```python
from build123d import *

# Parameters (mm, degrees)
TRAY_START                        = 4.75
SKETCH1_W                         = 36.8
SKETCH1_H                         = 53.4
TRAY_DEPTH                        = 2.89
GROOVE_START                      = 7.14
SKETCH2_W                         = 34.6
SKETCH2_H                         = 53.2
GROOVE_DEPTH                      = 0.6
GROOVE_START_2                    = 6.6
SKETCH3_W                         = 34.6
SKETCH3_H                         = 10.45
GROOVE_PROTECTION_BOARD_END_DEPTH = 0.55
S1_S3_START                       = 4.65
SKETCH4_W                         = 9.25
SKETCH4_H                         = 6.5
SKETCH4_W_2                       = 9.05
S1_S3_AND_PLUGS_DEPTH             = 3.09
J4_START                          = 4.65
SKETCH5_W                         = 17.5
SKETCH5_H                         = 6
J4_AND_ITS_FLEX_DEPTH             = 3.09
ARM_START                         = 4.75
SKETCH6_W                         = 8
SKETCH6_H                         = 14.2
ARM_DEPTH                         = 1.5
BOARD_START                       = 1.6
SKETCH7_R                         = 2
BOARD_SCREW_FOOT_DEPTH            = 3.16
BOARD_START_2                     = 1.5
SKETCH8_R                         = 1.1
BOARD_SCREW_HOLE_DEPTH            = 6.24
BOARD_START_3                     = 5.94
SKETCH9_R                         = 1.95
BOARD_SCREW_COUNTERBORE_DEPTH     = 1.8
MIC_START                         = 1.8
SKETCH10_R                        = 1.5
MIC_TUBE_DEPTH                    = 2.96
MIC_START_2                       = 1.7
SKETCH11_R                        = 0.5
MIC_BORE_DEPTH                    = 4.3
MIC_START_3                       = 5
SKETCH12_W                        = 3.68
SKETCH12_H                        = 1
MIC_DUCT_DEPTH                    = 1
SNAP_START                        = -3
SNAP_DEPTH                        = 6


with BuildPart() as part:
    # Sketch1 → Tray (new body)
    with BuildSketch(Plane(origin=(0, 0, 0), x_dir=(1, 0, 0), z_dir=(0, 1, 0)).offset(TRAY_START)):
        with Locations((0, 5.95)):
            Rectangle(SKETCH1_W, SKETCH1_H)
    extrude(amount=TRAY_DEPTH)

    # Sketch2 → Groove (cut)
    with BuildSketch(Plane(origin=(0, 0, 0), x_dir=(1, 0, 0), z_dir=(0, 1, 0)).offset(GROOVE_START)):
        with Locations((0, 5.95)):
            Rectangle(SKETCH2_W, SKETCH2_H)
    extrude(amount=GROOVE_DEPTH, mode=Mode.SUBTRACT)

    # Sketch3 → Groove, protection-board end (cut)
    with BuildSketch(Plane(origin=(0, 0, 0), x_dir=(1, 0, 0), z_dir=(0, 1, 0)).offset(GROOVE_START_2)):
        with Locations((0, 27.325)):
            Rectangle(SKETCH3_W, SKETCH3_H)
    extrude(amount=GROOVE_PROTECTION_BOARD_END_DEPTH, mode=Mode.SUBTRACT)

    # Sketch4 → S1-S3 and plugs (cut)
    with BuildSketch(Plane(origin=(0, 0, 0), x_dir=(1, 0, 0), z_dir=(0, 1, 0)).offset(S1_S3_START)):
        with Locations((-13.825, 1.5)):
            Rectangle(SKETCH4_W, SKETCH4_H)
        with Locations((13.925, 20.57)):
            Rectangle(SKETCH4_W_2, SKETCH4_H)
        with Locations((13.825, -17.5)):
            Rectangle(SKETCH4_W, SKETCH4_H)
    extrude(amount=S1_S3_AND_PLUGS_DEPTH, mode=Mode.SUBTRACT)

    # Sketch5 → J4 and its flex (cut)
    with BuildSketch(Plane(origin=(0, 0, 0), x_dir=(1, 0, 0), z_dir=(0, 1, 0)).offset(J4_START)):
        with Locations((-0.35, 29.8)):
            Rectangle(SKETCH5_W, SKETCH5_H)
    extrude(amount=J4_AND_ITS_FLEX_DEPTH, mode=Mode.SUBTRACT)

    # Sketch6 → Arm (add)
    with BuildSketch(Plane(origin=(0, 0, 0), x_dir=(1, 0, 0), z_dir=(0, 1, 0)).offset(ARM_START)):
        with Locations((0, -27.7)):
            Rectangle(SKETCH6_W, SKETCH6_H)
    extrude(amount=ARM_DEPTH)

    # Sketch7 → Board screw foot (add)
    with BuildSketch(Plane(origin=(0, 0, 0), x_dir=(1, 0, 0), z_dir=(0, 1, 0)).offset(BOARD_START)):
        with Locations(Location((-15.64, 6.64, 0), (0, 0, 289.091052509))):
            Circle(SKETCH7_R)
    extrude(amount=BOARD_SCREW_FOOT_DEPTH)

    # Sketch8 → Board screw hole (cut)
    with BuildSketch(Plane(origin=(0, 0, 0), x_dir=(1, 0, 0), z_dir=(0, 1, 0)).offset(BOARD_START_2)):
        with Locations(Location((-15.64, 6.64, 0), (0, 0, 90))):
            Circle(SKETCH8_R)
    extrude(amount=BOARD_SCREW_HOLE_DEPTH, mode=Mode.SUBTRACT)

    # Sketch9 → Board screw counterbore (cut)
    with BuildSketch(Plane(origin=(0, 0, 0), x_dir=(1, 0, 0), z_dir=(0, 1, 0)).offset(BOARD_START_3)):
        with Locations((-15.64, 6.64)):
            Circle(SKETCH9_R)
    extrude(amount=BOARD_SCREW_COUNTERBORE_DEPTH, mode=Mode.SUBTRACT)

    # Sketch10 → Mic tube (add)
    with BuildSketch(Plane(origin=(0, 0, 0), x_dir=(1, 0, 0), z_dir=(0, 1, 0)).offset(MIC_START)):
        with Locations(Location((15.32, 29.94, 0), (0, 0, 270))):
            Circle(SKETCH10_R)
    extrude(amount=MIC_TUBE_DEPTH)

    # Sketch11 → Mic bore (cut)
    with BuildSketch(Plane(origin=(0, 0, 0), x_dir=(1, 0, 0), z_dir=(0, 1, 0)).offset(MIC_START_2)):
        with Locations(Location((15.32, 29.94, 0), (0, 0, 270))):
            Circle(SKETCH11_R)
    extrude(amount=MIC_BORE_DEPTH, mode=Mode.SUBTRACT)

    # Sketch12 → Mic duct (cut)
    with BuildSketch(Plane(origin=(0, 0, 0), x_dir=(1, 0, 0), z_dir=(0, 1, 0)).offset(MIC_START_3)):
        with Locations((16.66, 29.94)):
            Rectangle(SKETCH12_W, SKETCH12_H)
    extrude(amount=MIC_DUCT_DEPTH, mode=Mode.SUBTRACT)

    # Sketch13 → Snap (add)
    with BuildSketch(Plane(origin=(0, 0, 0), x_dir=(0, 0, -1), z_dir=(1, 0, 0)).offset(SNAP_START)):
        Polygon((-33.6, 5.25), (-34.8, 5.25), (-34.8, 0.3), (-35.4, 0.3), (-35.4, -0.3), (-34.8, -1.3), (-33.6, -1.3), align=None)
    extrude(amount=SNAP_DEPTH)


solid = part.part
```
Input: part model. Units: mm. Frame: model coordinates. A direction names the side the tool comes from. Give positions to 0.01 mm unless a question says otherwise; leave off trailing zeros. Order: outer loops, then holes, each group sorted by start corner. A loop starts at its lowest first (then second) coordinate and runs counter-clockwise, first axis right, second up. Notation, with made-up numbers: M 61.5,-33 L 109.5,-33 A18 ccw 109.5,-4 Z; hole C -2,64.25 d9. An arc over 180 degrees is marked long. One line per question, with ' | ' between items.
1) Ray query, L1, parallel to X at y = 3.6, z = -29.94; L2, parallel to Y at x = -11, z = -20.5; L3, parallel to X at y = 6.45, z = -6.64. Return the intervals inside material, ascending.
Filled in:
L1: x = 13.82 to 14.82, 15.82 to 16.82 | L2: y = 4.75 to 7.14 | L3: x = -18.4 to -17.59, -13.69 to 18.4
2) Section A-A on x = -10. Output: boundary loops of the cut face in (y, z), and give its area (3 significant figures).
Filled in:
outline: M 4.75,-32.65 L 7.64,-32.65 L 7.64,-32.55 L 6.6,-32.55 L 6.6,-22.1 L 7.14,-22.1 L 7.14,-4.75 L 4.75,-4.75 Z; M 4.75,1.75 L 7.14,1.75 L 7.14,20.65 L 7.64,20.65 L 7.64,20.75 L 4.75,20.75 Z | area: 107 mm2
3) Section D-D on x = -6. Output: boundary loops of the cut face in (y, z).
Filled in:
outline: M 4.75,-26.8 L 6.6,-26.8 L 6.6,-22.1 L 7.14,-22.1 L 7.14,20.65 L 7.64,20.65 L 7.64,20.75 L 4.75,20.75 Z
4) Section B-B on z = -6.64. Output: boundary loops of the cut face in (x, y), and give its area (3 significant figures).
Filled in:
outline: M -18.4,4.75 L -17.64,4.75 L -17.64,1.6 L -16.74,1.6 L -16.74,5.94 L -17.59,5.94 L -17.59,7.64 L -18.4,7.64 Z; M -14.54,1.6 L -13.64,1.6 L -13.64,4.75 L 18.4,4.75 L 18.4,7.64 L 17.3,7.64 L 17.3,7.14 L -13.69,7.14 L -13.69,5.94 L -14.54,5.94 Z | area: 87.3 mm2
5) Contact query for flat-ended pins moving along their axis: P1, Ø4, axis at x = -11.5, z = 23, coming from the +Y side; P2, Ø0.8, axis at y = 5.5, z = 31, coming from the +X side; P3, Ø3, axis at x = 14.5, z = -24.5, coming from the +Y side; P4, Ø0.5, axis at x = 16.5, z = -29.5, coming from the -Y side. Output: stop coordinate, or through.
Filled in:
P1: passes through | P2: stops at x = 4 | P3: stops at y = 6.6 | P4: stops at y = 1.8
6) Draft query along Z for faces 1 (the face through (-16.2, 1.6, -5.5)), 2 (the face through (-14, 6, -4.75)), 3 (the face through (0, 2, 33.6)). Return one class per face: pulls with the +Z half, pulls with the -Z half, needs draft (parallel to the pull), parting line crosses it, or undercut.
Filled in:
face 1: needs draft | face 2: undercut | face 3: pulls with the -Z half
7) Access query for faces 4 (the face through (0, 6.25, 28)), 5 (the face through (8.4, 6, -30)), 6 (the face through (0, 6.6, -26)). Directions: +Z, -Z, +X, -X, +Y, -Y. A direction counts if a zero-diameter tool reaches every point of the face in a straight line with its end or side. Return the directions, or none.
Filled in:
face 4: +Z, +X, -X, +Y | face 5: -Z, +Y, -Y | face 6: +Y
8) Section C-C on y = 4. Output: boundary loops of the cut face in (x, z), and give its area (3 significant figures).
Filled in:
outline: C -15.64,-6.64 d4; M -3,33.6 L 3,33.6 L 3,34.8 L -3,34.8 Z; C 15.32,-29.94 d3; hole C -15.64,-6.64 d2.2; hole C 15.32,-29.94 d1 | area: 22.2 mm2
